Autodesk Fusion 360 part; units mm, degrees
sketch "Sketch1" plane through (0, 0, 0) normal (0, 0, 1) x (1, 0, 0)
  circle A0 centre (30, 30) radius 7
  dimension "d1" = 14
extrude "Extrude1" add sketch "Sketch1" along normal blind 8
sketch "Sketch2" plane through (0, 0, 0) normal (0, 0, -1) x (1, 0, 0)
  circle A0 centre (30, -30) radius 7
  circle A1 centre (30, -30) radius 8
  dimension "d4" = 16
extrude "Extrude2" add sketch "Sketch2" along normal blind 2 contours A0 | A1
sketch "Sketch3" plane through (0, 0, 8) normal (0, 0, 1) x (-1, 0, 0)
  circle A0 centre (-30, -30) radius 7
  circle A1 centre (-30, -30) radius 2.5
  circle A2 centre (-30, -30) radius 1.5
  circle A3 centre (-30, -30) radius 6
  circle A4 centre (-30, -30) radius 0.5
  circle A5 centre (-30, -30) radius 5
  dimension "d7" = 5
  dimension "d8" = 3
  dimension "d9" = 12
  dimension "d10" = 1
  dimension "d13" = 10
extrude "Extrude3" cut sketch "Sketch3" against normal blind 16 contours A4
extrude "Extrude4" cut sketch "Sketch3" against normal blind 1 contours A3
chamfer "Chamfer1" distance 2.5 distance2 1 1 edges at (34.6616, 31.8081, 8) measured on face at (26.5186, 30.2484, 8)
chamfer "Chamfer2" distance 1 distance2 1 1 edges at (30.4662, 29.8192, 8) measured on face at (28.1756, 30.1242, 8)
sketch "Sketch4" plane through (0, 0, -2) normal (0, 0, -1) x (1, 0, 0)
  circle A0 centre (30, -30) radius 0.5
  circle A1 centre (30, -30) radius 8
  circle A2 centre (30, -30) radius 5
  dimension "d20" = 10
chamfer "Chamfer3" distance 4.5 distance2 8.5 1 edges at (30.4662, 30.1808, -2) measured on face at (35.4684, 30.4223, -2)
Model file for the job. Use its own axes, mm. A direction names the side the tool comes from. Round coordinates to 2 decimals unless told otherwise and drop trailing zeros. Write each loop counter-clockwise with the first axis right and the second up, starting at its lowest first coordinate (ties: lowest second). Pieces come first, ordered by that corner, then holes. Notation, with made-up numbers: M 43.25,49 L 82.25,49 A14 ccw 82.25,66 Z; hole C 5,-18 d11. An arc over 180 degrees is marked long. Put each result on its own line as item: value.
Item 1: Cut at C-C (x = 23.75). List the corners of the cut face in (y, z), and give its area (3 significant figures).
Responses:
outline: M 25.01,-2 L 34.99,-2 L 34.99,0 L 33.15,0 L 33.15,8 L 26.85,8 L 26.85,0 L 25.01,0 Z
area: 70.4 mm²
Item 2: Mould opens along Y. For faces 1 (the flat face through (29.9, 35.2, -2)), 2 (the cylindrical face through (36.466, 32.681, 3.944)), 3 (the cylindrical face through (30.4, 29.7, 6.8)) say: +Y half, -Y half, draft (parallel to the pull), parting line (faces both ways), or undercut.
Responses:
face 1: draft
face 2: parting line
face 3: undercut
Item 3: Tool access for faces 4 (the flat face through (36, 32, 8)), 5 (the flat face through (34, 26, 7)): list every direction of +Z, -Z, +X, -X, +Y, -Y with a clear straight run to the whole face (end or side of a thin tool).
Responses:
face 4: +Z, +X, -X, +Y, -Y
face 5: +Z
Item 4: Probe L1, parallel to Y at x = 30, z = 7.3; L2, parallel to Y at x = 30, z = 6.75; L3, parallel to X at y = 31.75, z = 3.5. List the from-to ranges inside material, lowest first. Write a range as from..to.
Responses:
L1: 23..24, 25.75..29.2, 30.8..34.25, 36..37
L2: 23..29.5, 30.5..37
L3: 23.22..28.86, 31.14..36.78
Item 5: Flat gauge pins, fed straight in: P1, Ø3, axis at x = 34.5, z = 6, coming from the +Y side; P2, Ø1, axis at y = 32.5, z = 7, coming from the +X side; P3, Ø4, axis at x = 34, z = 3, coming from the +Y side. Where does each tip first touch, or does it go through?
Responses:
P1: y = 36.32
P2: x = 36.71
P3: y = 36.71
Item 6: Cut at D-D (z = 3.5). List the corners of the cut face in (x, y).
Responses:
outline: C 30,30 d14; hole C 30,30 d4.18
